Source: CAD feature listing. Evaluate the final solid. Frame: model axes, mm. Face numbers are marked on the shaded views. Coordinates: 2 decimals unless noted, no trailing zeros. Order: outer loops, then holes, each group sorted by start corner. A loop starts at its lowest first (then second) coordinate and runs counter-clockwise, first axis right, second up.
Item 1: Contact query for flat-ended pins moving along their axis: P1, Ø1, axis at x = 3.5, y = 6.5, coming from the +Z side; P2, Ø1.5, axis at x = -47.5, y = 7.5, coming from the +Z side; P3, Ø4, axis at y = 5.5, z = 40, coming from the -X side. Output: stop coordinate, or through.
Item 2: Ray query, line 1 (X direction, y = 3, z = -14); line 2 (X direction, y = 3, z = 26). Return the intervals inside material, ascending.
Item 3: Section A-A on y = 4.5. Return the cut outline in (x, z), then the cut area to 3 significant figures.
Item 4: Section B-B on x = -21. Return the cut outline in (y, z), then the cut area to 3 significant figures.
Item 5: Section C-C on z = 47. Return the cut outline in (x, y).
Item 6: Mould query, pull axis Z, two halves, no side actions, for the marked faces 1, 2 and 3. Classes: released by +Z, released by -Z, zero draft, split by the parting line, or undercut.
from build123d import *

# Parameters (mm, degrees)
BOSS_EXTRUDE2_DEPTH = 11


with BuildPart() as part:
    # aula 4 → Boss-Extrude2 (new body)
    with BuildSketch(Plane(origin=(0, 0, 0), x_dir=(1, 0, 0), z_dir=(0, 1, 0))):
        with BuildLine():
            Line((0, 0), (0, 60))
            Line((0, 60), (60, 60))
            Line((60, 60), (60, -60))
            ThreePointArc((60, -60), (30, -90), (0, -60))
            Line((0, -60), (-60, -60))
            Line((-60, -60), (-60, -20))
            ThreePointArc((-60, -20), (-70, -10), (-60, 0))
            Line((-60, 0), (0, 0))
        make_face()
    extrude(amount=BOSS_EXTRUDE2_DEPTH)


solid = part.part
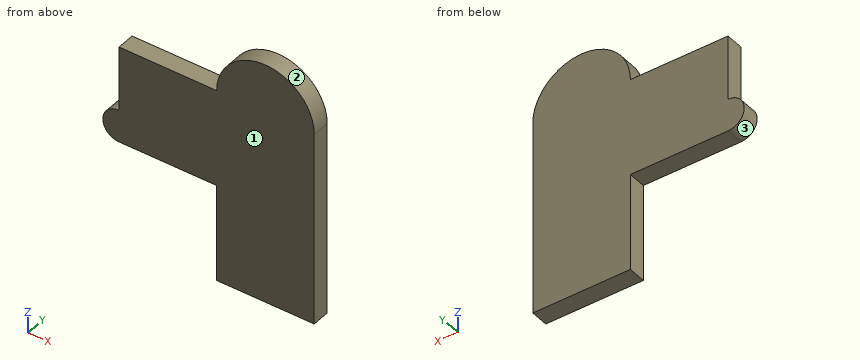
Answer list:
1. P1: stops at z = 74.97
1. P2: stops at z = 60
1. P3: stops at x = -60
2. line 1: x = 0 to 60
2. line 2: x = -60 to 60
3. outline: (-60, 0) - (0, 0) - (0, -60) - (60, -60) - (60, 60) arc R30 ccw to (0, 60) - (-60, 60) - (-60, 20) arc R10 ccw to start
3. area: 12,400 mm2
4. outline: (0, 0) - (11, 0) - (11, 60) - (0, 60) - close
4. area: 660 mm2
5. outline: (-60, 0) - (60, 0) - (60, 11) - (-60, 11) - close
6. face 1: zero draft
6. face 2: released by +Z
6. face 3: split by the parting line
